Answer from the drawing. Dimensions are ordinates in mm from the lowest x, y and z of the part. A direction names the side the tool comes from. Coordinates: 2 decimals unless noted, no trailing zeros. Loops run counter-clockwise (first coordinate to the right, second up) from the corner with the lowest first, then second, coordinate; pieces in that order, holes last.
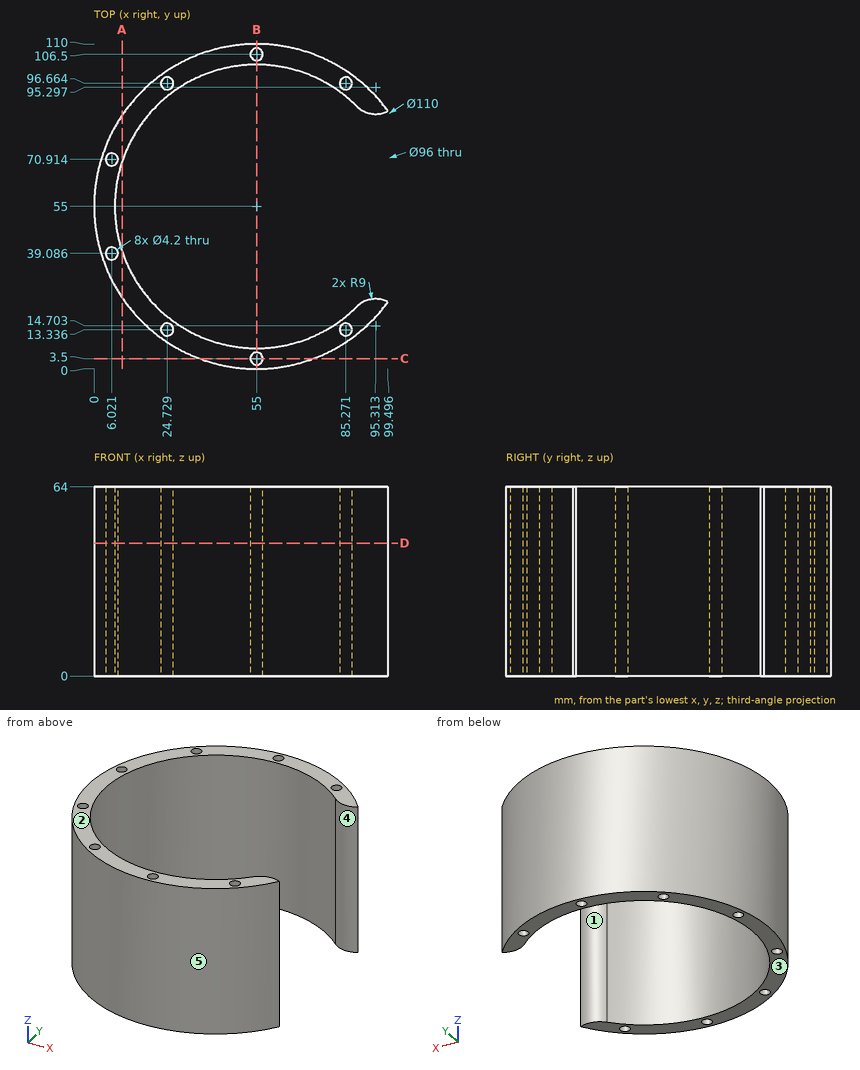
Item 1: A cutting plane is placed at B-B on x = 55. Determine the outline of the cut face in (y, z).
Numbers:
outline: (0, 0) - (1.4, 0) - (1.4, 64) - (0, 64) - close; (5.6, 0) - (7, 0) - (7, 64) - (5.6, 64) - close; (103, 0) - (104.4, 0) - (104.4, 64) - (103, 64) - close; (108.6, 0) - (110, 0) - (110, 64) - (108.6, 64) - close
Item 2: A cutting plane is placed at A-A on x = 9.5. Determine the outline of the cut face in (y, z), then the cut area to 3 significant figures.
Numbers:
outline: (24.1, 0) - (39.71, 0) - (39.71, 64) - (24.1, 64) - close; (70.29, 0) - (85.9, 0) - (85.9, 64) - (70.29, 64) - close
area: 2,000 mm2
Item 3: Given pin 1 (4 mm diameter, centred on x = 85.27, y = 96.66, fed in from -Z); pin 2 (12 mm diameter, centred on y = 86.5, z = 14, fed in from -X); pin 3 (10 mm diameter, centred on x = 57.5, z = 8, fed in from -Y); pin 4 (5 mm diameter, centred on x = 19, z = 6.5, fed in from +Y), each flat-ended and moving along its own axis, determine where each tip first touches the part or whether it passes through.
Numbers:
pin 1: passes through
pin 2: stops at x = 6.27
pin 3: stops at y = 0
pin 4: stops at y = 98.62
Item 4: Find the intervals of material crossed by line 1 along Y through (x, z) = (4.5, 37.5) (1 decimal); line 2 along Y through (x, z) = (56, 43) (1 decimal); line 3 along Y through (x, z) = (72.5, 45) (1 decimal), in increasing order.
Numbers:
line 1: y = 33.2 to 37.6, 40.5 to 69.5, 72.4 to 76.8
line 2: y = 0 to 1.7, 5.3 to 7, 103 to 104.7, 108.3 to 110
line 3: y = 2.9 to 10.3, 99.7 to 107.1
Item 5: A cutting plane is placed at C-C on y = 3.5. Determine the outline of the cut face in (x, z).
Numbers:
outline: (35.69, 0) - (52.9, 0) - (52.9, 64) - (35.69, 64) - close; (57.1, 0) - (74.31, 0) - (74.31, 64) - (57.1, 64) - close
Item 6: Determine the mould class of the marked faces 3, 4 and 5 for opening direction X: released by +X, released by -X, zero draft, split by the parting line, or undercut.
Numbers:
face 3: zero draft
face 4: undercut
face 5: split by the parting line
Item 7: Which of the six approach directions +Z, -Z, +X, -X, +Y, -Y give full straight-line access (tool end or side, diameter ignored) to the marked faces 1 and 2?
Numbers:
face 1: +Z, -Z
face 2: +Z, +X, -X, +Y, -Y
Item 8: A cutting plane is placed at D-D on z = 45. Give the number of separate pieces and of enclosed holes in the cut face, then the cut area to 3 significant figures.
Numbers:
separate pieces: 1
enclosed holes: 8
area: 1,680 mm2
